from build123d import *
from OCP.BRepFilletAPI import BRepFilletAPI_MakeChamfer

# Parameters (mm, degrees)
BOSS_EXTRUDE1_DEPTH = 200
SKETCH2_R           = 1.75
CUT_EXTRUDE1_DEPTH  = 10
SKETCH3_R           = 3
CUT_EXTRUDE2_DEPTH  = 4
CHAMFER1_SIZE       = 0.5
CHAMFER1_SIZE2      = 1.743707222
FILLET1_R           = 0.5


with BuildPart() as part:
    # Sketch1 → Boss-Extrude1 (new body)
    with BuildSketch(Plane(origin=(0, 0, 0), x_dir=(0, 0, -1), z_dir=(1, 0, 0))):
        Polygon((-0.5, 6), (4, 6), (4, -6), (-0.5, -6), (-0.5, -4.25), (-2.5, -4.25), (-2.5, -6), (-4, -6), (-4, 6), (-2.5, 6), (-2.5, 4.25), (-0.5, 4.25), align=None)
    extrude(amount=BOSS_EXTRUDE1_DEPTH)

    # Sketch2 → Cut-Extrude1 (cut)
    with BuildSketch(Plane.XY.offset(4)):
        with Locations((13, 0)):
            Circle(SKETCH2_R)
        with Locations((38, 0)):
            Circle(SKETCH2_R)
        with Locations((63, 0)):
            Circle(SKETCH2_R)
        with Locations((88, 0)):
            Circle(SKETCH2_R)
        with Locations((113, 0)):
            Circle(SKETCH2_R)
        with Locations((138, 0)):
            Circle(SKETCH2_R)
        with Locations((163, 0)):
            Circle(SKETCH2_R)
        with Locations((188, 0)):
            Circle(SKETCH2_R)
        with Locations((213, 0)):
            Circle(SKETCH2_R)
        with Locations((238, 0)):
            Circle(SKETCH2_R)
        with Locations((263, 0)):
            Circle(SKETCH2_R)
        with Locations((288, 0)):
            Circle(SKETCH2_R)
        with Locations((313, 0)):
            Circle(SKETCH2_R)
        with Locations((338, 0)):
            Circle(SKETCH2_R)
        with Locations((363, 0)):
            Circle(SKETCH2_R)
        with Locations((388, 0)):
            Circle(SKETCH2_R)
    extrude(amount=-CUT_EXTRUDE1_DEPTH, mode=Mode.SUBTRACT)

    # Sketch3 → Cut-Extrude2 (cut)
    with BuildSketch(Plane.XY.offset(4)):
        with Locations((13, 0)):
            Circle(SKETCH3_R)
        with Locations((38, 0)):
            Circle(SKETCH3_R)
        with Locations((63, 0)):
            Circle(SKETCH3_R)
        with Locations((88, 0)):
            Circle(SKETCH3_R)
        with Locations((113, 0)):
            Circle(SKETCH3_R)
        with Locations((138, 0)):
            Circle(SKETCH3_R)
        with Locations((163, 0)):
            Circle(SKETCH3_R)
        with Locations((188, 0)):
            Circle(SKETCH3_R)
        with Locations((213, 0)):
            Circle(SKETCH3_R)
        with Locations((238, 0)):
            Circle(SKETCH3_R)
        with Locations((263, 0)):
            Circle(SKETCH3_R)
        with Locations((288, 0)):
            Circle(SKETCH3_R)
        with Locations((313, 0)):
            Circle(SKETCH3_R)
        with Locations((338, 0)):
            Circle(SKETCH3_R)
        with Locations((363, 0)):
            Circle(SKETCH3_R)
        with Locations((388, 0)):
            Circle(SKETCH3_R)
    extrude(amount=-CUT_EXTRUDE2_DEPTH, mode=Mode.SUBTRACT)

    # Chamfer1: one chamfer whose edges measure the first distance from different faces: ONE call of the kernel's chamfer builder (chamfer() names one face for all edges)
    chamfer1_edges_1 = [part.edges().sort_by_distance(p)[0] for p in [
        (100, -4.25, 0.5),
        (100, -4.25, 2.5),
    ]]
    chamfer1_side_1 = [part.faces().sort_by_distance(p)[0] for p in [
        (100, -4.25, 1.5),
    ]]
    chamfer1_edges_2 = [part.edges().sort_by_distance(p)[0] for p in [
        (100, 4.25, 2.5),
        (100, 4.25, 0.5),
    ]]
    chamfer1_side_2 = [part.faces().sort_by_distance(p)[0] for p in [
        (100, 4.25, 1.5),
    ]]
    chamfer1 = BRepFilletAPI_MakeChamfer(part.part.solid().wrapped)
    for e in chamfer1_edges_1:
        chamfer1.Add(CHAMFER1_SIZE, CHAMFER1_SIZE2, e.wrapped, chamfer1_side_1[0].wrapped)  # the first distance lies on this face
    for e in chamfer1_edges_2:
        chamfer1.Add(CHAMFER1_SIZE, CHAMFER1_SIZE2, e.wrapped, chamfer1_side_2[0].wrapped)  # the first distance lies on this face
    add(Compound.cast(chamfer1.Shape()), mode=Mode.REPLACE)

    # Fillet1
    fillet1_edges = [part.edges().sort_by_distance(p)[0] for p in [
        (200, -6, -1.75),
        (200, 0, -4),
        (200, 6, -1.75),
        (200, 6, 3.25),
        (200, 0, 4),
        (200, -6, 3.25),
        (0, -6, 3.25),
        (0, -6, -1.75),
        (0, 0, -4),
        (0, 6, -1.75),
        (0, 6, 3.25),
        (0, 0, 4),
        (100, -4.25, 1),
        (100, -4.25, 2),
        (100, 4.25, 2),
        (100, 4.25, 1),
        (100, -6, 4),
        (100, 6, 4),
        (100, -6, -4),
        (100, 6, -4),
    ]]
    fillet(fillet1_edges, radius=FILLET1_R)


solid = part.part
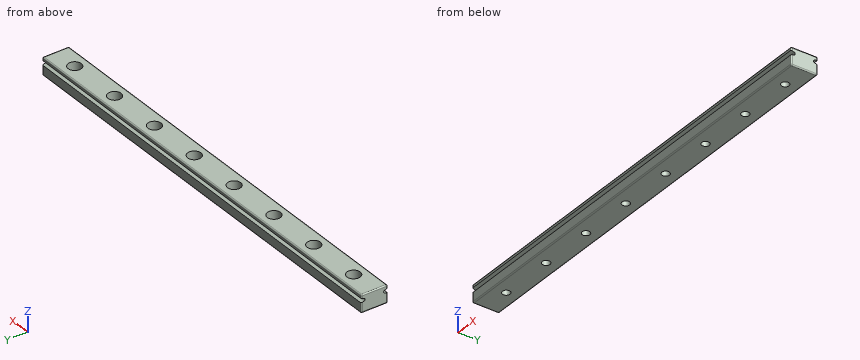
Check sheet for the modelled part. Datum: model origin and axes. Units: mm. Give positions to 0.01 mm unless a question says otherwise; leave off trailing zeros. Write item = value, one per line.
Item 1: Gauge pin test, flat end, axial feed: pin 1 (5.5 mm diameter, centred on x = 63, y = 0, fed in from +Z). Record the tip position at first contact, or that the pin passes through.
Output:
pin_1 = 0
Item 2: Sectioned sample at B-B on z = -1.75. Count the separate pieces of the cut face and the enclosed holes in it, and give its area (3 significant figures).
Output:
separate_pieces = 1
enclosed_holes = 8
area = 2,320 mm^2
Item 3: Scan lines: probe 1 along Y at (x, z) = (138, 2.55); probe 2 along Y at (x, z) = (63, -1.4); probe 3 along Z at (x, y) = (144.5, 5.25). Record each from-to range of solid material in increasing order. Write a range as from..to.
Output:
probe_1 = -6..-3, 3..6
probe_2 = -6..-1.75, 1.75..6
probe_3 = -4..0.71, 2.29..4
